```python
from build123d import *

# Parameters (mm, degrees)
F0_W           = 76.2
F0_H           = 25.4
F1_DEPTH       = 6.35
F3_D           = 3.175
F3_CBORE_D     = 6.35
F3_CBORE_DEPTH = 3.175
F4_W           = 38.1
F4_H           = 25.4
F6_W           = 38.1
F6_H           = 12.7
F8_W           = 38.1
F8_H           = 12.7
F9_DEPTH       = 38.1
F11_D          = 25.4


with BuildPart() as f1:
    # F0 (on Front) → F1 (new body)
    with BuildSketch(Plane.XZ):
        with Locations((38.1, 12.7)):
            Rectangle(F0_W, F0_H)
    extrude(amount=F1_DEPTH)

    # F3 (through all)
    with Locations(Plane.XZ.offset(6.35)):
        with Locations((6.35, 12.7), (69.85, 12.7)):
            CounterBoreHole(F3_D / 2, F3_CBORE_D / 2, F3_CBORE_DEPTH)

    # F4 (on face) → F7 section 0
    with BuildSketch(Plane.XZ.offset(6.35)):
        with Locations((38.1, 12.7)):
            Rectangle(F4_W, F4_H)
    # F6 (on offset) → F7 section 1
    with BuildSketch(Plane.XZ.offset(82.55)):
        with Locations((38.1, 12.7)):
            Rectangle(F6_W, F6_H)
    loft()

    # F8 (on face) → F9 (join)
    with BuildSketch(Plane.XZ.offset(82.55)):
        with Locations((38.1, 12.7)):
            Rectangle(F8_W, F8_H)
    extrude(amount=F9_DEPTH)

    # F11 (through all)
    with Locations(Plane(origin=(0, 0, 6.35), x_dir=(1, 0, 0), z_dir=(0, 0, -1))):
        with Locations((38.1, 101.6279906034)):
            Hole(F11_D / 2)


solid = f1.part
```
For this review, take the finished solid that the model builds, in its own axes (mm). A direction names the side the tool comes from. Coordinates: 2 decimals unless noted, no trailing zeros. Write each loop counter-clockwise with the first axis right and the second up, starting at its lowest first coordinate (ties: lowest second). Pieces come first, ordered by that corner, then holes.
(1) For pin 1 Ø10 at (x, y) = (35.5, -68.5) entering from +Z; pin 2 Ø11.5 at (x, y) = (29.5, -102.5) entering from -Z; pin 3 Ø12 at (x, z) = (57, 20) entering from +Y; pin 4 Ø3 at (x, z) = (7, 13) entering from -Y (3 decimals), all flat-tipped, find the tip position at first contact; note any pin that passes through.
(2) Wall thickness on probe 1 along Z at (x, y) = (69.85, -4.65) (3 decimals); probe 2 along Z at (x, y) = (69.85, -1.9); probe 3 along X at (y, z) = (-17.5, 11.75): over which ranges is each line inside the solid? List them lowest first.
(3) The part is to be moulded in two halves that separate along Z. For faces 5 (the face through (37.83, -44.98, 3.22)), 6 (the face through (66.5, -6.35, 12.9)), 7 (the face through (8, -3.175, 11)), say which applies: +Z half, -Z half, draft (parallel to the pull), parting line (faces both ways), or undercut.
(4) Add section A-A on x = 38.1. Give the boundary of the cut face in (y, z).
(5) Add section B-B on z = 12.7. Count the separate pieces of the cut face and the enclosed holes in it, then the cut area to 3 significant figures.
(6) Add section C-C on y = -96.5. Give the boundary of the cut face in (x, z).
(7) Add section D-D on x = 53. Give the boundary of the cut face in (y, z).
(8) Tool access review of faces 1 (the face through (57.15, -50, 13)), 2 (the face through (12, -6.35, 13)), 3 (the face through (67.33, -4.78, 10.77)), 4 (the face through (37.8, -88.6, 19.05)): name each direction out of +Z, -Z, +X, -X, +Y, -Y from which nothing blocks a thin tool from reaching the whole face with its end or side.
Answer sheet:
1. pin 1: stops at z = 20.64
1. pin 2: stops at z = 6.35
1. pin 3: stops at y = 0
1. pin 4: stops at y = -3.175
2. probe 1: z = 0 to 9.525, 15.875 to 25.4
2. probe 2: z = 0 to 11.11, 14.29 to 25.4
2. probe 3: x = 19.05 to 57.15
3. face 5: -Z half
3. face 6: draft
3. face 7: undercut
4. outline: (-120.65, 6.35) - (-114.33, 6.35) - (-114.33, 19.05) - (-120.65, 19.05) - close; (-88.93, 6.35) - (-82.55, 6.35) - (-6.35, 0) - (0, 0) - (0, 25.4) - (-6.35, 25.4) - (-82.55, 19.05) - (-88.93, 19.05) - close
5. separate pieces: 3
5. enclosed holes: 1
5. area: 4,270 mm2
6. outline: (19.05, 6.35) - (26.48, 6.35) - (26.48, 19.05) - (19.05, 19.05) - close; (49.72, 6.35) - (57.15, 6.35) - (57.15, 19.05) - (49.72, 19.05) - close
7. outline: (-120.65, 6.35) - (-82.55, 6.35) - (-6.35, 0) - (0, 0) - (0, 25.4) - (-6.35, 25.4) - (-82.55, 19.05) - (-120.65, 19.05) - close
8. face 1: +Z, -Z, +X, -Y
8. face 2: +Z, -Z, -X, -Y
8. face 3: -Y
8. face 4: +Z, +X, -X, -Y
